Source: CAD feature listing. Evaluate the final solid. Frame: model axes, mm. A direction names the side the tool comes from. Coordinates: 2 decimals unless noted, no trailing zeros. Order: outer loops, then holes, each group sorted by start corner. A loop starts at its lowest first (then second) coordinate and runs counter-clockwise, first axis right, second up.
Item 1: Ray query, line 1 (Z direction, x = -38, y = 4); line 2 (X direction, y = -42.5, z = 3); line 3 (Y direction, x = -17.5, z = 5.25). Return the intervals inside material, ascending.
Item 2: Section C-C on y = -3.5. Return the cut outline in (x, z).
Item 3: Reachability of faces 4 (the cylindrical face through (47.388, -41.887, 3.549)), 5 (the flat face through (0, -9, 2)) from +Z, -Z, +X, -X, +Y, -Y: full face, straight path, thin tool, end or side. Return the list, or none.
Item 4: Mould query, pull axis X, two halves, no side actions, for faces 1 (the flat face through (-47, -11, 7)), 2 (the cylindrical face through (49.97, -39.94, 6.49)), 3 (the cylindrical face through (-48.11, -13.23, 3.55)). Classes: released by +X, released by -X, zero draft, split by the parting line, or undercut.
Item 5: Section B-B on x = 20. Return the cut outline in (y, z).
Item 6: Section A-A on z = 4.5. State how many separate pieces and enclosed holes the cut face has, then the cut area to 3 significant figures.
Item 7: Contact query for flat-ended pins moving along their axis: P1, Ø3, axis at x = -32, z = 6, coming from the -Y side; P2, Ø4, axis at x = -25.5, z = 4.5, coming from the -Y side; P3, Ø22.5, axis at x = 18.5, y = -9, coming from the +Z side. Output: stop coordinate, or through.
from build123d import *

# Parameters (mm, degrees)
SKETCH1_W           = 100.85
SKETCH1_H           = 70.53
BOSS_EXTRUDE1_DEPTH = 2
SKETCH6_W           = 104.85
SKETCH6_H           = 74.53
BOSS_EXTRUDE3_DEPTH = 2
SKETCH3_R           = 2.5
BOSS_EXTRUDE2_DEPTH = 5
FILLET1_SIZE        = 1.5
FILLET1_SIZE_2      = 4


with BuildPart() as part:
    # Sketch1 → Boss-Extrude1 (new body)
    with BuildSketch(Plane.XY):
        with Locations((0.782139599, -9.454393248)):
            Rectangle(SKETCH1_W, SKETCH1_H)
    extrude(amount=BOSS_EXTRUDE1_DEPTH)

    # Sketch6 → Boss-Extrude3 (add)
    with BuildSketch(Plane.XY.offset(2)):
        with Locations((0.782139599, -9.454393248)):
            Rectangle(SKETCH6_W, SKETCH6_H)
    extrude(amount=-BOSS_EXTRUDE3_DEPTH)

    # Sketch3 → Boss-Extrude2 (add)
    with BuildSketch(Plane.XY.offset(2)):
        with Locations((-29.192860401, 22.360606752)):
            Circle(SKETCH3_R)
    boss_extrude2 = extrude(amount=BOSS_EXTRUDE2_DEPTH)

    # Sketch5 → Tap Drill for M3x0.5 Tap1 (revolve, cut)
    with BuildSketch(Plane(origin=(-29.192860401, 22.360606752, 7), x_dir=(0, -1, 0), z_dir=(1, 0, 0))):
        Polygon((0, 0), (0, 10.751075774), (1.25, 10), (1.25, 0), align=None)
    tap_drill_for_m3x0_5_tap1 = revolve(axis=Axis((-29.192860401, 22.360606752, 13.35), (0, 0, -1)), mode=Mode.SUBTRACT)

    # Sketch-Pattern1: Boss-Extrude2, Tap Drill for M3x0.5 Tap1 at 4 more places
    with Locations((-17.86, -34.92, 0), (13.94, -37.51, 0), (77.82, -64.41, 0), (62.15, 0.23, 0)):
        add(boss_extrude2)
        add(tap_drill_for_m3x0_5_tap1, mode=Mode.SUBTRACT)

    # Fillet1
    # an asymmetric fillet: 4, 1.5 mm, written as the material it adds along each edge
    with BuildSketch(Plane(origin=(-29.192860401, 22.360606752, 2), x_dir=(1, 0, 0), z_dir=(0, -1, 0))) as fillet1_piece_1:
        with BuildLine():
            Bezier((2.5 + FILLET1_SIZE, 0), (2.5, 0), (2.5, FILLET1_SIZE_2), weights=[1, 0.707106781, 1])
            Line((2.5, FILLET1_SIZE_2), (2.5, 0))
            Line((2.5, 0), (2.5 + FILLET1_SIZE, 0))
        make_face()
    revolve(axis=Axis((-29.192860401, 22.360606752, 2), (0, 0, 1)))
    with BuildSketch(Plane(origin=(-47.052860401, -12.559393248, 2), x_dir=(1, 0, 0), z_dir=(0, -1, 0))) as fillet1_piece_2:
        with BuildLine():
            Bezier((2.5 + FILLET1_SIZE, 0), (2.5, 0), (2.5, FILLET1_SIZE_2), weights=[1, 0.707106781, 1])
            Line((2.5, FILLET1_SIZE_2), (2.5, 0))
            Line((2.5, 0), (2.5 + FILLET1_SIZE, 0))
        make_face()
    revolve(axis=Axis((-47.052860401, -12.559393248, 2), (0, 0, 1)))
    with BuildSketch(Plane(origin=(-15.252860401, -15.149393248, 2), x_dir=(1, 0, 0), z_dir=(0, -1, 0))) as fillet1_piece_3:
        with BuildLine():
            Bezier((2.5 + FILLET1_SIZE, 0), (2.5, 0), (2.5, FILLET1_SIZE_2), weights=[1, 0.707106781, 1])
            Line((2.5, FILLET1_SIZE_2), (2.5, 0))
            Line((2.5, 0), (2.5 + FILLET1_SIZE, 0))
        make_face()
    revolve(axis=Axis((-15.252860401, -15.149393248, 2), (0, 0, 1)))
    with BuildSketch(Plane(origin=(48.627139599, -42.049393248, 2), x_dir=(1, 0, 0), z_dir=(0, -1, 0))) as fillet1_piece_4:
        with BuildLine():
            Bezier((2.5 + FILLET1_SIZE, 0), (2.5, 0), (2.5, FILLET1_SIZE_2), weights=[1, 0.707106781, 1])
            Line((2.5, FILLET1_SIZE_2), (2.5, 0))
            Line((2.5, 0), (2.5 + FILLET1_SIZE, 0))
        make_face()
    revolve(axis=Axis((48.627139599, -42.049393248, 2), (0, 0, 1)))
    with BuildSketch(Plane(origin=(32.957139599, 22.590606752, 2), x_dir=(1, 0, 0), z_dir=(0, -1, 0))) as fillet1_piece_5:
        with BuildLine():
            Bezier((2.5 + FILLET1_SIZE, 0), (2.5, 0), (2.5, FILLET1_SIZE_2), weights=[1, 0.707106781, 1])
            Line((2.5, FILLET1_SIZE_2), (2.5, 0))
            Line((2.5, 0), (2.5 + FILLET1_SIZE, 0))
        make_face()
    revolve(axis=Axis((32.957139599, 22.590606752, 2), (0, 0, 1)))


solid = part.part
Answer list:
1. line 1: z = 0 to 2
1. line 2: x = 45.65 to 47.46, 49.79 to 51.6
1. line 3: y = -16.3 to -13.99
2. outline: (-51.64, 0) - (53.21, 0) - (53.21, 2) - (-51.64, 2) - close
3. face 4: +Z, -Z
3. face 5: +Z
4. face 1: zero draft
4. face 2: split by the parting line
4. face 3: undercut
5. outline: (-46.72, 0) - (27.81, 0) - (27.81, 2) - (-46.72, 2) - close
6. separate pieces: 5
6. enclosed holes: 5
6. area: 82.4 mm2
7. P1: stops at y = 20.23
7. P2: stops at y = 20.3
7. P3: stops at z = 2
